Work out the finished part from the listing and answer in its coordinate system (mm). A direction names the side the tool comes from. Round coordinates to 2 decimals unless told otherwise and drop trailing zeros. Order: outer loops, then holes, each group sorted by start corner. A loop starts at its lowest first (then second) coordinate and runs counter-clockwise, first axis right, second up. Notation, with made-up numbers: (53.5, 44.5) -> (89.5, 44.5) arc R23 cw to (89.5, 69.5) -> close; hole circle Ø4 at (-16.75, 28). An arc over 180 degrees is marked (long way). Use one line per item in the form item = value.
```python
from build123d import *

# Parameters (mm, degrees)
BOSS_EXTRUDE1_DEPTH = 48
SKETCH3_R           = 11
BOSS_EXTRUDE2_DEPTH = 2
SKETCH4_R           = 2.5
BOSS_EXTRUDE3_DEPTH = 22
CUT_EXTRUDE2_START  = -15
CUT_EXTRUDE2_DEPTH  = 15


with BuildPart() as part:
    # Sketch2 → Boss-Extrude1 (new body)
    with BuildSketch(Plane.XY):
        Polygon((5.65, 0), (36.65, 0), (42.3, 5.65), (42.3, 36.65), (36.65, 42.3), (5.65, 42.3), (0, 36.65), (0, 5.65), align=None)
    extrude(amount=BOSS_EXTRUDE1_DEPTH)

    # Sketch3 → Boss-Extrude2 (add)
    with BuildSketch(Plane.XY.offset(48)):
        with Locations((21.15, 21.15)):
            Circle(SKETCH3_R)
    extrude(amount=BOSS_EXTRUDE2_DEPTH)

    # Sketch4 → Boss-Extrude3 (add)
    with BuildSketch(Plane.XY.offset(50)):
        with Locations((21.15, 21.15)):
            Circle(SKETCH4_R)
    extrude(amount=BOSS_EXTRUDE3_DEPTH)

    # Sketch5 → Cut-Extrude2 (cut)
    with BuildSketch(Plane.XY.offset(72).offset(CUT_EXTRUDE2_START)):
        with BuildLine():
            ThreePointArc((19.65, 23.15), (20.359430585, 23.521708245), (21.15, 23.65))
            ThreePointArc((21.15, 23.65), (21.940569415, 23.521708245), (22.65, 23.15))
            Line((22.65, 23.15), (25.205995561, 23.15))
            Line((25.205995561, 23.15), (25.205995561, 25.058533995))
            Line((25.205995561, 25.058533995), (17.955034994, 25.058533995))
            Line((17.955034994, 25.058533995), (17.955034994, 23.15))
            Line((17.955034994, 23.15), (19.65, 23.15))
        make_face()
        with BuildLine():
            ThreePointArc((22.65, 23.15), (21.940569415, 23.521708245), (21.15, 23.65))
            Line((21.15, 23.65), (21.15, 23.15))
            Line((21.15, 23.15), (22.65, 23.15))
        make_face()
        with BuildLine():
            Line((21.15, 23.15), (21.15, 23.65))
            ThreePointArc((21.15, 23.65), (20.359430585, 23.521708245), (19.65, 23.15))
            Line((19.65, 23.15), (21.15, 23.15))
        make_face()
    extrude(amount=CUT_EXTRUDE2_DEPTH, mode=Mode.SUBTRACT)


solid = part.part
```
Item 1: The part is cut by section D-D, the plane y = 21.15. Give the vertices of the cut face in (x, z), and give its area (3 significant figures).
Findings:
outline = (0, 0) -> (42.3, 0) -> (42.3, 48) -> (32.15, 48) -> (32.15, 50) -> (23.65, 50) -> (23.65, 72) -> (18.65, 72) -> (18.65, 50) -> (10.15, 50) -> (10.15, 48) -> (0, 48) -> close
area = 2,180 mm^2
Item 2: Flat-ended cylindrical pins translate along their axes: P1, Ø8, axis at x = 36.5, y = 23.5, coming from the +Z side; P2, Ø1.5, axis at x = 22, z = 61, coming from the +Y side; P3, Ø6, axis at x = 5.5, z = 51.5, coming from the +Y side. Find the tip coordinate at first contact, or state that the pin passes through.
Findings:
P1 = 48
P2 = 23.15
P3 = through
Item 3: The part is cut by section B-B, the plane z = 15.5. Give the vertices of the cut face in (x, y), and give its area (3 significant figures).
Findings:
outline = (0, 5.65) -> (5.65, 0) -> (36.65, 0) -> (42.3, 5.65) -> (42.3, 36.65) -> (36.65, 42.3) -> (5.65, 42.3) -> (0, 36.65) -> close
area = 1,730 mm^2
Item 4: Consider line 1 along Z through (x, y) = (23, 9); line 2 along Z through (x, y) = (19, 12.5); line 3 along Y through (x, z) = (37, 18.5). Determine where each line is inside the solid, lowest interval first.
Findings:
line_1 = 0 to 48
line_2 = 0 to 50
line_3 = 0.35 to 41.95
Item 5: The part is cut by section A-A, the plane x = 21.15. Give the vertices of the cut face in (y, z).
Findings:
outline = (0, 0) -> (42.3, 0) -> (42.3, 48) -> (32.15, 48) -> (32.15, 50) -> (23.65, 50) -> (23.65, 57) -> (23.15, 57) -> (23.15, 72) -> (18.65, 72) -> (18.65, 50) -> (10.15, 50) -> (10.15, 48) -> (0, 48) -> close
Item 6: The part is cut by section C-C, the plane y = 27.5. Give the vertices of the cut face in (x, z).
Findings:
outline = (0, 0) -> (42.3, 0) -> (42.3, 48) -> (30.13, 48) -> (30.13, 50) -> (12.17, 50) -> (12.17, 48) -> (0, 48) -> close
Item 7: For faces 1 (the cylindrical face through (20.61, 18.71, 60.85)), 2 (the flat face through (21, 23.15, 64)), 3 (the flat face through (2.79, 2.86, 23.66)), determine the directions among +Z, -Z, +X, -X, +Y, -Y from which every point of the face is accessible in a straight line to the end or side of a thin tool.
Findings:
face_1 = +Z
face_2 = +Z, +X, -X, +Y
face_3 = +Z, -Z, -X, -Y
